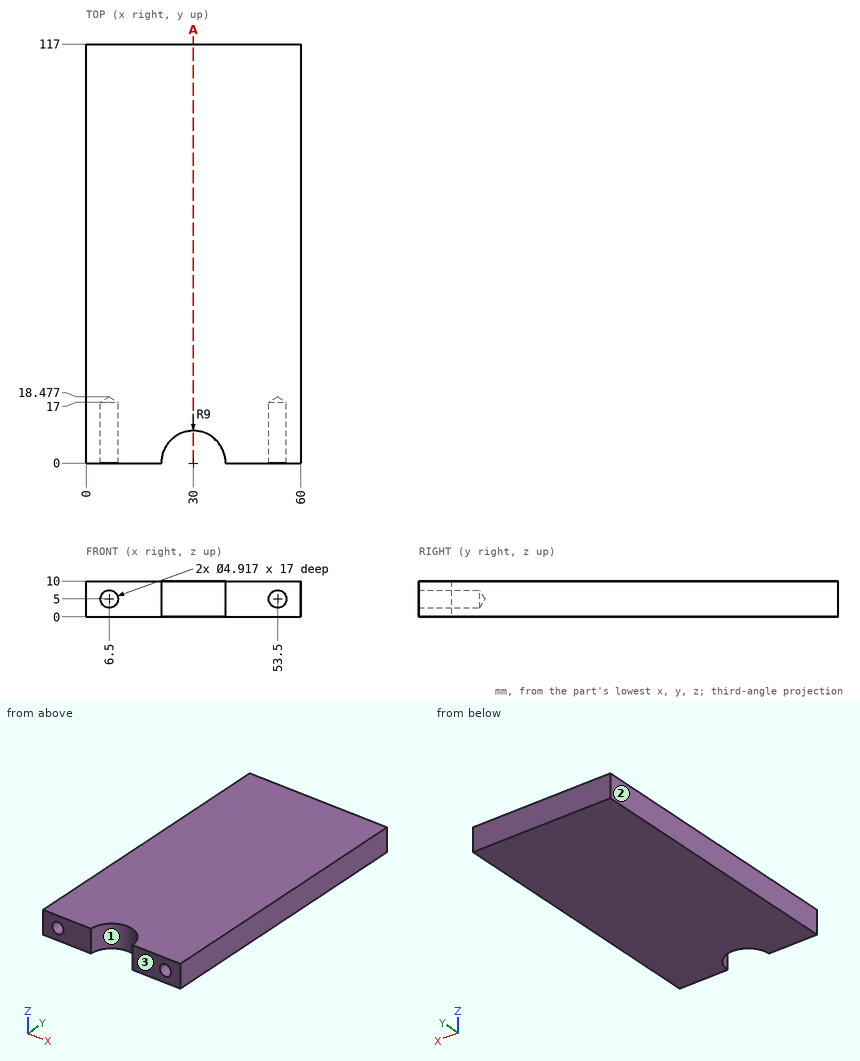
Answer from the drawing. Dimensions are ordinates in mm from the lowest x, y and z of the part. Give positions to 0.01 mm unless a question says otherwise; leave off trailing zeros. Order: outer loops, then holes, each group sorted by start corner. A loop starts at its lowest first (then second) coordinate and runs counter-clockwise, first axis right, second up. Notation, with made-up numbers: (75.5, 3.5) -> (127.5, 3.5) arc R31 ccw to (127.5, 29.5) -> close; hole circle Ø8 at (33, 42.25). An arc over 180 degrees is marked (long way). One line per item, written item: value. Start each with the question number.
(1) For a pull along X with two mould halves and no side action, classify the marked faces 1, 2 and 3 as released by +X, released by -X, zero draft, split by the parting line, or undercut.
(2) Straight lines are drawn through the part: L1, parallel to X at y = 6, z = 5; L2, parallel to Z at x = 6.5, y = 7.5; L3, parallel to X at y = 7.75, z = 5 (1 decimal). For each, find the intervals that lie inside material, in ascending order.
(3) The part is cut by section A-A (x = 30). Determine the outline of the cut face in (y, z), and give its area (3 significant figures).
Taken from the geometry:
1. face 1: undercut
1. face 2: released by -X
1. face 3: zero draft
2. L1: 0 to 4.04, 8.96 to 23.29, 36.71 to 51.04, 55.96 to 60
2. L2: 0 to 2.54, 7.46 to 10
2. L3: 0 to 4, 9 to 25.4, 34.6 to 51, 56 to 60
3. outline: (9, 0) -> (117, 0) -> (117, 10) -> (9, 10) -> close
3. area: 1,080 mm^2
